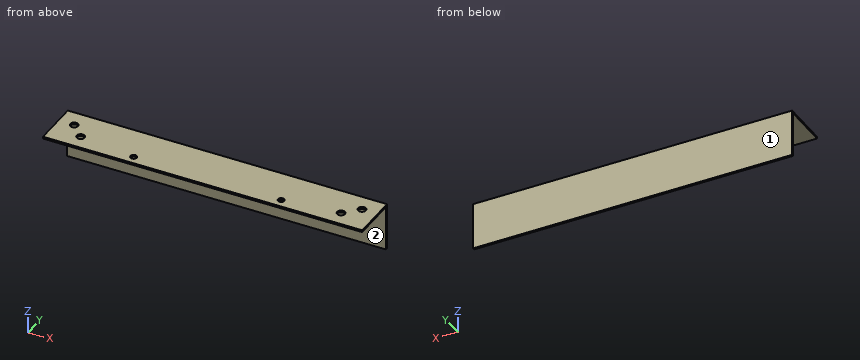
from build123d import *

# Parameters (mm, degrees)
PAD007_DEPTH      = 129.237
PAD007_DEPTH_BACK = 129.237
SKETCH017_R       = 2.54
SKETCH017_R_2     = 3.175
POCKET007_DEPTH   = 1.6002


with BuildPart() as pocket007:
    # Sketch016 → Pad007 (new body, two sides)
    with BuildSketch(Plane(origin=(0, -90.5002, -38.1), x_dir=(0, 1, 0), z_dir=(1, 0, 0))) as pad007_sk:
        Polygon((0, 0), (38.1, 0), (38.1, -1.6002), (1.6002, -1.6002), (1.6002, -38.1), (0, -38.1), align=None)
    extrude(amount=PAD007_DEPTH)
    extrude(pad007_sk.sketch, amount=-PAD007_DEPTH_BACK)

    # Sketch017 → Pocket007 (cut)
    with BuildSketch(Plane(origin=(0, -90.5002, -39.7002), x_dir=(0, 1, 0), z_dir=(0, 0, -1))):
        with Locations((30.734, 59.69)):
            Circle(SKETCH017_R)
        with Locations((30.734, -59.69)):
            Circle(SKETCH017_R)
        with Locations((25.4, -105.4372)):
            Circle(SKETCH017_R_2)
        with Locations((14.3002, -116.537)):
            Circle(SKETCH017_R_2)
        with Locations((14.3002, 116.537)):
            Circle(SKETCH017_R_2)
        with Locations((25.4, 105.4372)):
            Circle(SKETCH017_R_2)
    extrude(amount=-POCKET007_DEPTH, mode=Mode.SUBTRACT)


with BuildPart() as part_mirroring005:
    # Part__Mirroring005: instance of Pocket007
    add(pocket007.part.mirror(Plane(origin=(0, 0, 0), x_dir=(1, 0, 0), z_dir=(0, 1, 0))))


solid = part_mirroring005.part
Work out the finished part from the listing and answer in its coordinate system (mm). Face numbers are marked on the shaded views. A direction names the side the tool comes from. Give positions to 0.01 mm unless a question says otherwise; leave off trailing zeros. Loops run counter-clockwise (first coordinate to the right, second up) from the corner with the lowest first, then second, coordinate; pieces in that order, holes last. Notation, with made-up numbers: (51.25, 30.25) -> (95.25, 30.25) arc R29 cw to (95.25, 68.25) -> close; hole circle Ø11 at (38.25, 78). An arc over 180 degrees is marked (long way). Use a Markdown table: item, result. Add a question column.
1) The part is cut by section B-B, the plane x = -59.69. Determine the outline of the cut face in (y, z).
2) Consider line 1 along X through (y, z) = (76.2, -39.1); line 2 along Z through (x, y) = (29, 88); line 3 along Y through (x, z) = (20, -55.5). Determine where each line is inside the solid, lowest interval first.
3) Each of these flat-tipped pins is pushed along its axis until it touches: P1, Ø1.5, axis at x = 100, z = -62.5, coming from the -Y side; P2, Ø6.5, axis at x = -59.69, y = 59.77, coming from the +Z side; P3, Ø10, axis at x = 89.5, y = 73.5, coming from the -Z side; P4, Ø5, axis at x = 116.537, y = 76.2, coming from the -Z side. Where does it stop, or does it pass through?
4) The part is cut by section D-D, the plane x = 45.5. Determine the outline of the cut face in (y, z).
5) The part is cut by section C-C, the plane z = -59. Determine the outline of the cut face in (x, y).
6) Which of the six approach directions +Z, -Z, +X, -X, +Y, -Y give full straight-line access (tool end or side, diameter ignored) to the marked faces 1 and 2?
7) The part is cut by section A-A, the plane y = 76.2. Determine the outline of the cut face in (x, z), plus the area to 3 significant figures.
Reported:
| question | item | result |
|---|---|---|
| 1 | outline | (52.4, -39.7) -> (57.23, -39.7) -> (57.23, -38.1) -> (52.4, -38.1) -> close; (62.31, -39.7) -> (88.9, -39.7) -> (88.9, -76.2) -> (90.5, -76.2) -> (90.5, -38.1) -> (62.31, -38.1) -> close |
| 2 | line 1 | x = -129.24 to -119.71, -113.36 to 113.36, 119.71 to 129.24 |
| 2 | line 2 | z = -39.7 to -38.1 |
| 2 | line 3 | y = 88.9 to 90.5 |
| 3 | P1 | stops at y = 88.9 |
| 3 | P2 | stops at z = -38.1 |
| 3 | P3 | stops at z = -39.7 |
| 3 | P4 | passes through |
| 4 | outline | (52.4, -39.7) -> (88.9, -39.7) -> (88.9, -76.2) -> (90.5, -76.2) -> (90.5, -38.1) -> (52.4, -38.1) -> close |
| 5 | outline | (-129.24, 88.9) -> (129.24, 88.9) -> (129.24, 90.5) -> (-129.24, 90.5) -> close |
| 6 | face 1 | +Z, -Z, +X, -X, +Y |
| 6 | face 2 | -Z, +X, -X, -Y |
| 7 | outline | (-129.24, -39.7) -> (-119.71, -39.7) -> (-119.71, -38.1) -> (-129.24, -38.1) -> close; (-113.36, -39.7) -> (113.36, -39.7) -> (113.36, -38.1) -> (-113.36, -38.1) -> close; (119.71, -39.7) -> (129.24, -39.7) -> (129.24, -38.1) -> (119.71, -38.1) -> close |
| 7 | area | 393 mm^2 |
